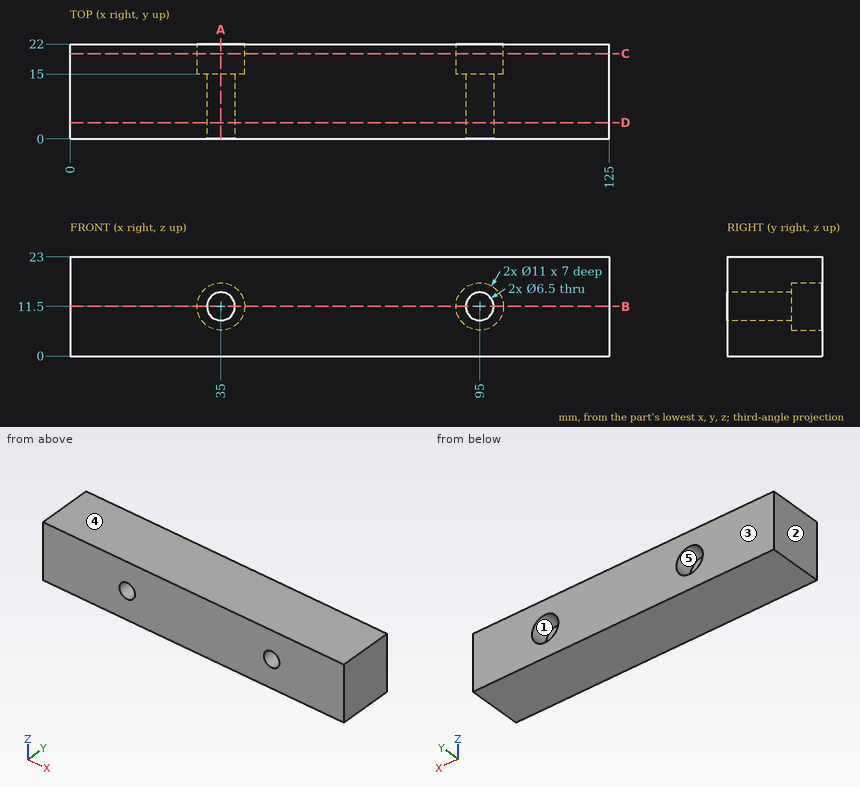
Here's the drawing with two shaded views (mm, measured from the low corner). I have some questions. A direction names the side the tool comes from. Coordinates: 2 decimals unless noted, no trailing zeros. Write each loop counter-clockwise with the first axis right and the second up, starting at its lowest first coordinate (ties: lowest second). Pieces come first, ordered by that corner, then holes. Notation, with made-up numbers: M 20,-33.75 L 47,-33.75 A28 cw 47,-13.75 Z; hole C 38,-6 d8. An arc over 180 degrees is marked long. Write item = value, one per line. Start each with the question number.
Q1. Thinking about a two-plate mould opening in X: for the marked faces 1, 2 and 3, which applies, released by +X, released by -X, zero draft, split by the parting line, or undercut?
Q2. If we section it at C-C, the plane y = 19.75: Write out the boundary of the cut face in (x, z).
Q3. If I drill on L1, parallel to X at y = 11.5, z = 11.5; L2, parallel to Z at x = 95, y = 18.5; L3, parallel to Z at x = 95, y = 11.5, over which ranges is the centre line in solid material (lowest first)? Write a range as [from, to].
Q4. If we section it at D-D, the plane y = 3.75: Write out the boundary of the cut face in (x, z), then the cut area to 3 significant figures.
Q5. If we section it at B-B, the plane z = 11.5: Write out the boundary of the cut face in (x, y), then the cut area to 3 significant figures.
Q6. On a 3-axis mill with a long thin cutter (end or side, diameter ignored), from which of +Z, -Z, +X, -X, +Y, -Y can I reach the whole of each face in a straight line? I mean the marked faces 4 and 5. Say none if no direction works.
Q7. I'm going to push a flat-ended pin straight in: pin 1 (10 mm diameter, centred on x = 35, z = 11.5, fed in from +Y). Where does the tip first touch, or does it pass through?
Q8. If we section it at A-A, the plane x = 35: Write out the boundary of the cut face in (y, z).
Check sheet entries:
q1.face_1 = undercut
q1.face_2 = released by -X
q1.face_3 = zero draft
q2.outline = M 0,0 L 125,0 L 125,23 L 0,23 Z; hole C 35,11.5 d11; hole C 95,11.5 d11
q3.L1 = [0, 31.75], [38.25, 91.75], [98.25, 125]
q3.L2 = [0, 6], [17, 23]
q3.L3 = [0, 8.25], [14.75, 23]
q4.outline = M 0,0 L 125,0 L 125,23 L 0,23 Z; hole C 35,11.5 d6.5; hole C 95,11.5 d6.5
q4.area = 2,810 mm²
q5.outline = M 0,0 L 31.75,0 L 31.75,15 L 29.5,15 L 29.5,22 L 0,22 Z; M 38.25,0 L 91.75,0 L 91.75,15 L 89.5,15 L 89.5,22 L 40.5,22 L 40.5,15 L 38.25,15 Z; M 98.25,0 L 125,0 L 125,22 L 100.5,22 L 100.5,15 L 98.25,15 Z
q5.area = 2,400 mm²
q6.face_4 = +Z, +X, -X, +Y, -Y
q6.face_5 = +Y
q7.pin_1 = 15
q8.outline = M 0,0 L 22,0 L 22,6 L 15,6 L 15,8.25 L 0,8.25 Z; M 0,14.75 L 15,14.75 L 15,17 L 22,17 L 22,23 L 0,23 Z
